Answer from the drawing. Dimensions are ordinates in mm from the lowest x, y and z of the part. A direction names the side the tool comes from. Round coordinates to 2 decimals unless told otherwise and drop trailing zeros. Write each loop counter-clockwise with the first axis right and the second up, starting at its lowest first coordinate (ties: lowest second). Pieces come first, ordered by that corner, then holes. Notation, with made-up numbers: (4, 83) -> (39, 83) arc R24 cw to (39, 98) -> close; hole circle Ø7 at (79, -24). An arc over 180 degrees is marked (long way). Return JSON: item names as keys, results as strings. Group by question number.
(1) A cutting plane is placed at A-A on z = 51.75. Give the vertices of the cut face in (x, y), then the cut area to 3 significant figures.
(2) A cutting plane is placed at B-B on y = 10. Give the vertices of the cut face in (x, z).
(3) A cutting plane is placed at D-D on x = 33.5. Give the vertices of the cut face in (y, z).
(4) Straight lines are drawn through the part: line 1 (Y direction, x = 20.6, z = 51.75); line 2 (Y direction, x = 21, z = 51); line 3 (Z direction, x = 22, y = 13). For each, find the intervals that lie inside material, in ascending order.
(5) Given pin 1 (4 mm diameter, centred on y = 9.5, z = 47.5, fed in from +X); pin 2 (2 mm diameter, centred on y = 11.5, z = 51, fed in from +X); pin 3 (12 mm diameter, centred on y = 4.5, z = 21, fed in from -X); pin 4 (6 mm diameter, centred on y = 7, z = 3, fed in from -X), each flat-ended and moving along its own axis, determine where each tip first touches the part or whether it passes through.
(6) A cutting plane is placed at C-C on z = 36.5. Give the vertices of the cut face in (x, y), then the cut area to 3 significant figures.
(7) For the marked faces 1, 2 and 3, determine the directions among +Z, -Z, +X, -X, +Y, -Y from which every point of the face is accessible in a straight line to the end or side of a thin tool.
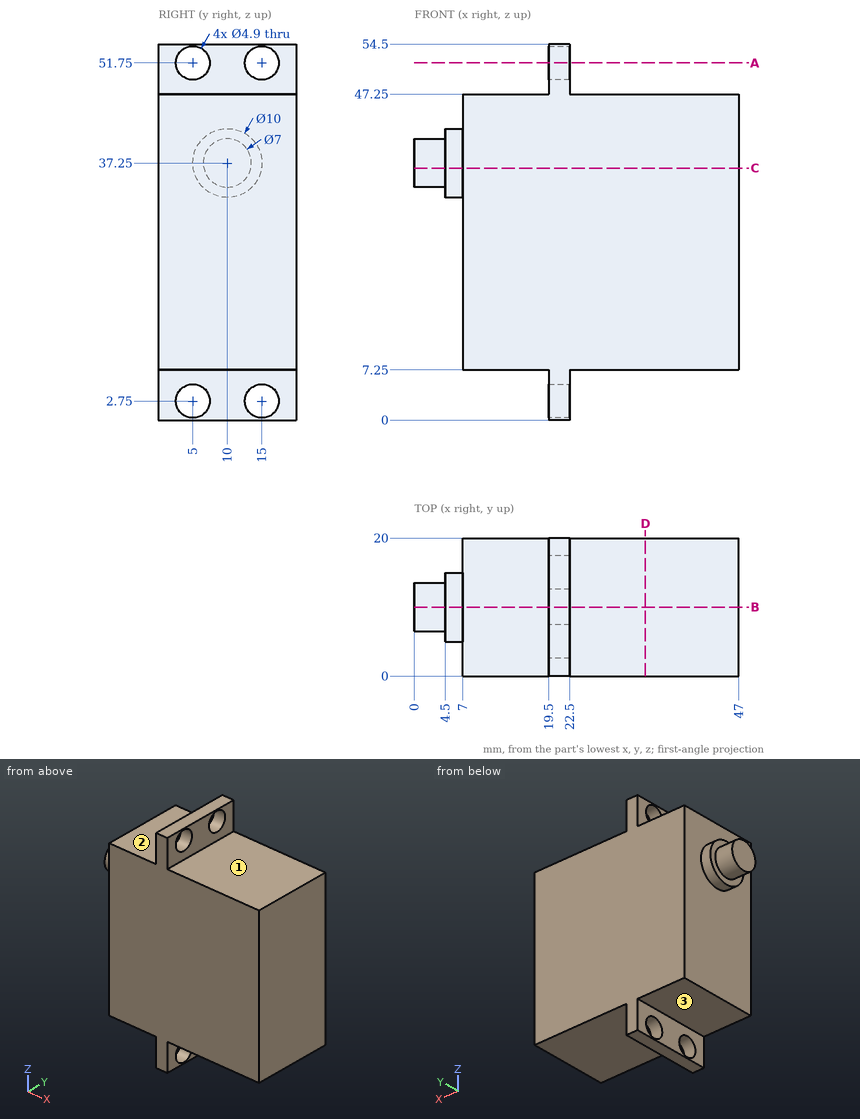
Checks:
{
 "1": {"outline": "(19.5, 0) -> (22.5, 0) -> (22.5, 2.55) -> (19.5, 2.55) -> close; (19.5, 7.45) -> (22.5, 7.45) -> (22.5, 12.55) -> (19.5, 12.55) -> close; (19.5, 17.45) -> (22.5, 17.45) -> (22.5, 20) -> (19.5, 20) -> close", "area": "30.6 mm^2"},
 "2": {"outline": "(0, 33.75) -> (4.5, 33.75) -> (4.5, 32.25) -> (7, 32.25) -> (7, 7.25) -> (19.5, 7.25) -> (19.5, 0) -> (22.5, 0) -> (22.5, 7.25) -> (47, 7.25) -> (47, 47.25) -> (22.5, 47.25) -> (22.5, 54.5) -> (19.5, 54.5) -> (19.5, 47.25) -> (7, 47.25) -> (7, 42.25) -> (4.5, 42.25) -> (4.5, 40.75) -> (0, 40.75) -> close"},
 "3": {"outline": "(0, 7.25) -> (20, 7.25) -> (20, 47.25) -> (0, 47.25) -> close"},
 "4": {"line 1": "y = 0 to 2.55, 7.45 to 12.55, 17.45 to 20", "line 2": "y = 0 to 2.67, 7.33 to 12.67, 17.33 to 20", "line 3": "z = 0 to 1.33, 4.17 to 50.33, 53.17 to 54.5"},
 "5": {"pin 1": "stops at x = 47", "pin 2": "stops at x = 22.5", "pin 3": "stops at x = 7", "pin 4": "stops at x = 19.5"},
 "6": {"outline": "(0, 6.58) -> (4.5, 6.58) -> (4.5, 5.06) -> (7, 5.06) -> (7, 0) -> (47, 0) -> (47, 20) -> (7, 20) -> (7, 14.94) -> (4.5, 14.94) -> (4.5, 13.42) -> (0, 13.42) -> close", "area": "855 mm^2"},
 "7": {"face 1": "+Z, +X, +Y, -Y", "face 2": "+Z, -X, +Y, -Y", "face 3": "-Z, -X, +Y, -Y"}
}
